Can you work these out from the model? Positions are in its coordinate system, mm. Round coordinates to 2 decimals unless told otherwise and drop trailing zeros. Loops run counter-clockwise (first coordinate to the right, second up) from the corner with the lowest first, then second, coordinate; pieces in that order, holes last. Notation, with made-up numbers: (75, 29.5) - (133, 29.5) arc R29 ccw to (133, 51.5) - close; hole circle Ø10 at (23.25, 84.25). An arc over 180 degrees is marked (long way). Answer as CSV lines item,"result".
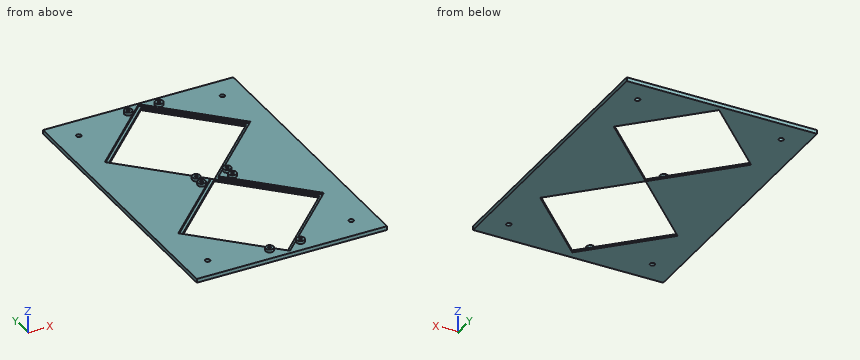
```python
from build123d import *

# Parameters (mm, degrees)
ESQUISSE1_W                          = 194
ESQUISSE1_H                          = 294
BOSS_EXTRU_1_DEPTH                   = 4
ESQUISSE2_R                          = 2.5
ENL_V_MAT_EXTRU_4_DEPTH              = 5
ENL_V_MAT_EXTRU_17_DEPTH             = 5
R_P_TITION_LIN_AIRE2_COUNT           = 2
R_P_TITION_LIN_AIRE2_PITCH           = 141.43
ESQUISSE5_R                          = 4
BOSS_EXTRU_2_DEPTH                   = 3
ESQUISSE6_R                          = 1.5
ENL_V_MAT_EXTRU_18_DEPTH             = 6
ESQUISSE7_R                          = 1.5
ENL_V_MAT_EXTRU_19_DEPTH             = 6
R_P_TITION_LIN_AIRE5_COUNT           = 2
R_P_TITION_LIN_AIRE5_PITCH           = 130.815
ESQUISSE10_R                         = 1.5
ENL_V_MAT_EXTRU_20_DEPTH             = 6
ESQUISSE9_R                          = 4
BOSS_EXTRU_3_DEPTH                   = 3
ESQUISSE11_R                         = 1.5
ENL_V_MAT_EXTRU_21_DEPTH             = 6
R_P_TITION_LIN_AIRE6_COUNT           = 2
R_P_TITION_LIN_AIRE6_PITCH           = 31.82
R_P_TITION_LIN_AIRE7_COUNT           = 2
R_P_TITION_LIN_AIRE7_PITCH           = 130.815
R_P_TITION_LIN_AIRE7_COPY_1_SKETCH_R = 4
R_P_TITION_LIN_AIRE7_COPY_1_DEPTH    = 3
R_P_TITION_LIN_AIRE7_COPY_2_SKETCH_R = 1.5
R_P_TITION_LIN_AIRE7_COPY_2_DEPTH    = 6
ENL_V_MAT_EXTRU_22_DEPTH             = 2
ENL_V_MAT_EXTRU_23_DEPTH             = 2
ENL_V_MAT_EXTRU_25_DEPTH             = 2
ENL_V_MAT_EXTRU_27_DEPTH             = 2
ENL_V_MAT_EXTRU_28_DEPTH             = 2
ENL_V_MAT_EXTRU_29_DEPTH             = 2
ENL_V_MAT_EXTRU_30_DEPTH             = 2
ENL_V_MAT_EXTRU_31_DEPTH             = 2
ESQUISSE23_W                         = 4
ESQUISSE23_H                         = 294
BOSS_EXTRU_4_DEPTH                   = 1
R_P_TITION_LIN_AIRE8_COUNT           = 2
R_P_TITION_LIN_AIRE8_PITCH           = 195
ESQUISSE24_W                         = 196
ESQUISSE24_H                         = 4
BOSS_EXTRU_5_DEPTH                   = 1
R_P_TITION_LIN_AIRE9_COUNT           = 2
R_P_TITION_LIN_AIRE9_PITCH           = 295


with BuildPart() as part:
    # Esquisse1 → Boss.-Extru.1 (new body)
    with BuildSketch(Plane.XY):
        with Locations((76.321557543, 133.418871343)):
            Rectangle(ESQUISSE1_W, ESQUISSE1_H)
    extrude(amount=BOSS_EXTRU_1_DEPTH)

    # Esquisse2 → Enl_v. mat.-Extru.4 (cut, through all)
    with BuildSketch(Plane.XY):
        with Locations((2.321557543, 257.418871343)):
            Circle(ESQUISSE2_R)
        with Locations((150.321557543, 257.418871343)):
            Circle(ESQUISSE2_R)
        with Locations((150.321557543, 9.418871343)):
            Circle(ESQUISSE2_R)
        with Locations((2.321557543, 9.418871343)):
            Circle(ESQUISSE2_R)
    extrude(amount=ENL_V_MAT_EXTRU_4_DEPTH, mode=Mode.SUBTRACT)

    # Esquisse4 → Enl_v. mat.-Extru.17 (cut, through all)
    with BuildSketch(Plane.XY.offset(4)):
        Polygon((76.321557543, 276.118871343), (5.610879425, 205.408193225), (76.321557543, 134.697515106), (147.032235662, 205.408193225), align=None)
    enl_v_mat_extru_17 = extrude(amount=-ENL_V_MAT_EXTRU_17_DEPTH, mode=Mode.SUBTRACT)

    # R_p_tition lin_aire2: Enl_v. mat.-Extru.17 ×2
    with Locations(*[(0, -i * R_P_TITION_LIN_AIRE2_PITCH, 0) for i in range(1, R_P_TITION_LIN_AIRE2_COUNT)]):
        add(enl_v_mat_extru_17, mode=Mode.SUBTRACT)

    # Esquisse5 → Boss.-Extru.2 (add)
    with BuildSketch(Plane.XY.offset(4)):
        with Locations((60.411654967, 270.815570484)):
            Circle(ESQUISSE5_R)
        with Locations((92.23146012, 270.815570484)):
            Circle(ESQUISSE5_R)
    boss_extru_2 = extrude(amount=BOSS_EXTRU_2_DEPTH)

    # Esquisse6 → Enl_v. mat.-Extru.18 (cut)
    with BuildSketch(Plane.XY.offset(7)):
        with Locations((60.411654967, 270.815570484)):
            Circle(ESQUISSE6_R)
    enl_v_mat_extru_18 = extrude(amount=-ENL_V_MAT_EXTRU_18_DEPTH, mode=Mode.SUBTRACT)

    # Esquisse7 → Enl_v. mat.-Extru.19 (cut)
    with BuildSketch(Plane.XY.offset(7)):
        with Locations((92.23146012, 270.815570484)):
            Circle(ESQUISSE7_R)
    extrude(amount=-ENL_V_MAT_EXTRU_19_DEPTH, mode=Mode.SUBTRACT)

    # R_p_tition lin_aire5: Boss.-Extru.2, Enl_v. mat.-Extru.18 ×2
    with Locations(*[(0, -i * R_P_TITION_LIN_AIRE5_PITCH, 0) for i in range(1, R_P_TITION_LIN_AIRE5_COUNT)]):
        add(boss_extru_2)
        add(enl_v_mat_extru_18, mode=Mode.SUBTRACT)

    # Esquisse10 → Enl_v. mat.-Extru.20 (cut)
    with BuildSketch(Plane.XY.offset(7)):
        with Locations((92.23146012, 140.000570484)):
            Circle(ESQUISSE10_R)
    extrude(amount=-ENL_V_MAT_EXTRU_20_DEPTH, mode=Mode.SUBTRACT)

    # Esquisse9 → Boss.-Extru.3 (add)
    with BuildSketch(Plane.XY.offset(4)):
        with Locations((92.23146012, 129.385570484)):
            Circle(ESQUISSE9_R)
    boss_extru_3 = extrude(amount=BOSS_EXTRU_3_DEPTH)

    # Esquisse11 → Enl_v. mat.-Extru.21 (cut)
    with BuildSketch(Plane.XY.offset(7)):
        with Locations((92.23146012, 129.385570484)):
            Circle(ESQUISSE11_R)
    enl_v_mat_extru_21 = extrude(amount=-ENL_V_MAT_EXTRU_21_DEPTH, mode=Mode.SUBTRACT)

    # R_p_tition lin_aire6: Boss.-Extru.3, Enl_v. mat.-Extru.21 ×2
    with Locations(*[(-i * R_P_TITION_LIN_AIRE6_PITCH, 0, 0) for i in range(1, R_P_TITION_LIN_AIRE6_COUNT)]):
        add(boss_extru_3)
        add(enl_v_mat_extru_21, mode=Mode.SUBTRACT)

    # R_p_tition lin_aire7: Boss.-Extru.3, Enl_v. mat.-Extru.21 ×2
    with Locations(*[(0, -i * R_P_TITION_LIN_AIRE7_PITCH, 0) for i in range(1, R_P_TITION_LIN_AIRE7_COUNT)]):
        add(boss_extru_3)
        add(enl_v_mat_extru_21, mode=Mode.SUBTRACT)

    # R_p_tition lin_aire7 copy 1 sketch → R_p_tition lin_aire7 copy 1 (add)
    with BuildSketch(Plane(origin=(-31.82, -130.815, 4), x_dir=(1, 0, 0), z_dir=(0, 0, 1))):
        with Locations((92.23146012, 129.385570484)):
            Circle(R_P_TITION_LIN_AIRE7_COPY_1_SKETCH_R)
    extrude(amount=R_P_TITION_LIN_AIRE7_COPY_1_DEPTH)

    # R_p_tition lin_aire7 copy 2 sketch → R_p_tition lin_aire7 copy 2 (cut)
    with BuildSketch(Plane(origin=(-31.82, -130.815, 7), x_dir=(1, 0, 0), z_dir=(0, 0, 1))):
        with Locations((92.23146012, 129.385570484)):
            Circle(R_P_TITION_LIN_AIRE7_COPY_2_SKETCH_R)
    extrude(amount=-R_P_TITION_LIN_AIRE7_COPY_2_DEPTH, mode=Mode.SUBTRACT)

    # Esquisse13 → Enl_v. mat.-Extru.22 (cut)
    with BuildSketch(Plane.XY.offset(4)):
        Polygon((76.321557543, 276.118871343), (147.032235662, 205.408193225), (149.153556006, 207.529513568), (78.442877887, 278.240191687), align=None)
    extrude(amount=-ENL_V_MAT_EXTRU_22_DEPTH, mode=Mode.SUBTRACT)

    # Esquisse14 → Enl_v. mat.-Extru.23 (cut)
    with BuildSketch(Plane.XY.offset(4)):
        Polygon((5.610879425, 205.408193225), (78.442877887, 278.240191687), (76.321557543, 280.36151203), (3.489559081, 207.529513568), align=None)
    extrude(amount=-ENL_V_MAT_EXTRU_23_DEPTH, mode=Mode.SUBTRACT)

    # Esquisse15 → Enl_v. mat.-Extru.25 (cut)
    with BuildSketch(Plane.XY.offset(4)):
        Polygon((76.325879425, 134.693193225), (3.489559081, 207.529513568), (1.368238738, 205.408193225), (74.204559081, 132.571872881), align=None)
    extrude(amount=-ENL_V_MAT_EXTRU_25_DEPTH, mode=Mode.SUBTRACT)

    # Esquisse16 → Enl_v. mat.-Extru.27 (cut)
    with BuildSketch(Plane.XY.offset(4)):
        Polygon((76.317235662, 134.693193225), (149.153556006, 207.529513568), (151.274876349, 205.408193225), (78.438556006, 132.571872881), align=None)
    extrude(amount=-ENL_V_MAT_EXTRU_27_DEPTH, mode=Mode.SUBTRACT)

    # Esquisse19 → Enl_v. mat.-Extru.28 (cut)
    with BuildSketch(Plane.XY.offset(4)):
        Polygon((74.204559081, 132.571872881), (5.610879425, 63.978193225), (3.489559081, 66.099513568), (72.083238738, 134.693193225), align=None)
    extrude(amount=-ENL_V_MAT_EXTRU_28_DEPTH, mode=Mode.SUBTRACT)

    # Esquisse20 → Enl_v. mat.-Extru.29 (cut)
    with BuildSketch(Plane.XY.offset(4)):
        Polygon((3.489559081, 66.099513568), (76.321557543, -6.732484894), (74.2002372, -8.853805238), (1.368238738, 63.978193225), align=None)
    extrude(amount=-ENL_V_MAT_EXTRU_29_DEPTH, mode=Mode.SUBTRACT)

    # Esquisse21 → Enl_v. mat.-Extru.30 (cut)
    with BuildSketch(Plane.XY.offset(4)):
        Polygon((74.2002372, -8.853805238), (147.032235662, 63.978193225), (149.153556006, 61.856872881), (76.321557543, -10.975125581), align=None)
    extrude(amount=-ENL_V_MAT_EXTRU_30_DEPTH, mode=Mode.SUBTRACT)

    # Esquisse22 → Enl_v. mat.-Extru.31 (cut)
    with BuildSketch(Plane.XY.offset(4)):
        Polygon((149.153556006, 61.856872881), (78.438556006, 132.571872881), (80.559876349, 134.693193225), (151.274876349, 63.978193225), align=None)
    extrude(amount=-ENL_V_MAT_EXTRU_31_DEPTH, mode=Mode.SUBTRACT)

    # Esquisse23 → Boss.-Extru.4 (add)
    with BuildSketch(Plane(origin=(173.321557543, 0, 0), x_dir=(0, 0, -1), z_dir=(1, 0, 0))):
        with Locations((-2, 133.418871343)):
            Rectangle(ESQUISSE23_W, ESQUISSE23_H)
    boss_extru_4 = extrude(amount=BOSS_EXTRU_4_DEPTH)

    # R_p_tition lin_aire8: Boss.-Extru.4 ×2
    with Locations(*[(-i * R_P_TITION_LIN_AIRE8_PITCH, 0, 0) for i in range(1, R_P_TITION_LIN_AIRE8_COUNT)]):
        add(boss_extru_4)

    # Esquisse24 → Boss.-Extru.5 (add)
    with BuildSketch(Plane(origin=(0, 280.418871343, 0), x_dir=(1, 0, 0), z_dir=(0, 1, 0))):
        with Locations((76.321557543, -2)):
            Rectangle(ESQUISSE24_W, ESQUISSE24_H)
    boss_extru_5 = extrude(amount=BOSS_EXTRU_5_DEPTH)

    # R_p_tition lin_aire9: Boss.-Extru.5 ×2
    with Locations(*[(0, -i * R_P_TITION_LIN_AIRE9_PITCH, 0) for i in range(1, R_P_TITION_LIN_AIRE9_COUNT)]):
        add(boss_extru_5)


solid = part.part
```
Q1. Imagine slicing it at A-A (x = 69). Write out the boundary of the cut face in (y, z), then the cut area to 3 significant figures.
Checks:
outline,"(-14.58, 0) - (0.59, 0) - (0.59, 2) - (-3.65, 2) - (-3.65, 4) - (-14.58, 4) - close; (127.37, 0) - (142.02, 0) - (142.02, 2) - (137.78, 2) - (137.78, 4) - (131.61, 4) - (131.61, 2) - (127.37, 2) - close; (268.8, 0) - (281.42, 0) - (281.42, 4) - (273.04, 4) - (273.04, 2) - (268.8, 2) - close"
area,"136 mm²"
Q2. I'm going to push flat-ended pins straight in: pin 1 Ø0.9 at (x, y) = (60, 129.5) entering from +Z; pin 2 Ø6 at (x, y) = (150.32, 257.42) entering from +Z; pin 3 Ø4.5 at (x, y) = (2.32, 257.42) entering from -Z. Where does each tip first touch, or does it pass through?
Checks:
pin 1,"z = 1"
pin 2,"z = 4"
pin 3,"through"
Q3. Imagine slicing it at C-C (z = 5.5). Count the separate pieces of the cut face and the enclosed holes in it, then the cut area to 3 significant figures.
Checks:
separate pieces,"8"
enclosed holes,"8"
area,"346 mm²"
Q4. If I drill on line 1 along Y through (x, z) = (133, 2.75); line 2 along Y through (x, z) = (105, 2.25); line 3 along Z through (x, y) = (137, 141), over which ranges is the centre line in solid material (lowest first)? Write a range as [from, to].
Checks:
line 1,"[-14.58, 45.7], [82.25, 187.13], [223.68, 281.42]"
line 2,"[-14.58, 17.7], [110.25, 159.13], [251.68, 281.42]"
line 3,"[0, 4]"
Q5. Imagine slicing it at B-B (y = 213). Write out the boundary of the cut face in (x, z), then the cut area to 3 significant figures.
Checks:
outline,"(-21.68, 0) - (13.2, 0) - (13.2, 2) - (8.96, 2) - (8.96, 4) - (-21.68, 4) - close; (139.44, 0) - (174.32, 0) - (174.32, 4) - (143.68, 4) - (143.68, 2) - (139.44, 2) - close"
area,"262 mm²"
Q6. Imagine slicing it at D-D (x = 25). Write out the boundary of the cut face in (y, z), then the cut area to 3 significant figures.
Checks:
outline,"(-14.58, 0) - (44.59, 0) - (44.59, 2) - (40.35, 2) - (40.35, 4) - (-14.58, 4) - close; (83.37, 0) - (186.02, 0) - (186.02, 2) - (181.78, 2) - (181.78, 4) - (87.61, 4) - (87.61, 2) - (83.37, 2) - close; (224.8, 0) - (281.42, 0) - (281.42, 4) - (229.04, 4) - (229.04, 2) - (224.8, 2) - close"
area,"840 mm²"
